from build123d import *

# Parameters (mm, degrees)
SKETCH_1_W          = 10
SKETCH_1_H          = 11.5
SKETCH_1_R          = 1.6
EXTRUDE_1_DEPTH     = 3
SKETCH_2_W          = 15
SKETCH_2_H          = 6
EXTRUDE_2_DEPTH     = 5
FILLET_1_R          = 1
SKETCH_3_W          = 5
SKETCH_3_H          = 5
EXTRUDE_3_DEPTH     = 2
SKETCH_4_W          = 5
SKETCH_4_H          = 3
EXTRUDE_4_DEPTH     = 19.5
SKETCH_5_W          = 5
SKETCH_5_H          = 3.5
EXTRUDE_5_DEPTH     = 3
SKETCH_6_W          = 3
SKETCH_6_H          = 8.5
EXTRUDE_6_DEPTH     = 3
EXTRUDE_7_DEPTH     = 1
SKETCH_8_W          = 3.5
SKETCH_8_H          = 21.5
EXTRUDE_8_DEPTH     = 1
SKETCH_9_W          = 3
SKETCH_9_H          = 8
EXTRUDE_9_DEPTH     = 3.5
EXTRUDE_10_REACH    = 29.208
SKETCH_10_W         = 2.5
SKETCH_10_H         = 3.5
EXTRUDE_11_REACH    = 29.208
SKETCH_11_W         = 3
SKETCH_11_H         = 4
SKETCH_12_W         = 1.5
SKETCH_12_H         = 1.2
CUT_EXTRUDE_1_DEPTH = 2
SKETCH_13_W         = 1
SKETCH_13_H         = 2.5
EXTRUDE_12_DEPTH    = 6.5
SKETCH_14_W         = 1.2
SKETCH_14_H         = 8
EXTRUDE_13_DEPTH    = 6.5
SKETCH_15_W         = 4
SKETCH_15_H         = 4
EXTRUDE_14_DEPTH    = 2.8
FILLET_2_R          = 1
CUT_EXTRUDE_2_REACH = 33.357
SKETCH_16_R         = 1.6
SKETCH_17_W         = 15
SKETCH_17_H         = 5
EXTRUDE_15_DEPTH    = 2
EXTRUDE_16_DEPTH    = 5.5
SKETCH_19_W         = 2
SKETCH_19_H         = 2.8
EXTRUDE_17_DEPTH    = 2
EXTRUDE_18_DEPTH    = 5.5
EXTRUDE_19_DEPTH    = 2.9
EXTRUDE_20_DEPTH    = 0.5
FILLET_3_R          = 2
SKETCH_23_W         = 14.9
SKETCH_23_H         = 1.5
EXTRUDE_21_DEPTH    = 0.5
SKETCH_24_W         = 3
SKETCH_24_H         = 2.8
EXTRUDE_22_DEPTH    = 5
EXTRUDE_23_DEPTH    = 3.2


with BuildPart() as part:
    # 草图1 → 凸台-拉伸1 (new body)
    with BuildSketch(Plane.XY):
        with Locations((1, 0.75)):
            Rectangle(SKETCH_1_W, SKETCH_1_H)
        Circle(SKETCH_1_R, mode=Mode.SUBTRACT)
    extrude(amount=EXTRUDE_1_DEPTH)

    # 草图2 → 凸台-拉伸2 (add)
    with BuildSketch(Plane.XY.offset(3)):
        with Locations((13.5, -2)):
            Rectangle(SKETCH_2_W, SKETCH_2_H)
    extrude(amount=-EXTRUDE_2_DEPTH)

    # 圆角1
    fillet_1_edges = [part.edges().sort_by_distance(p)[0] for p in [
        (-4, 0.75, 0),
    ]]
    fillet(fillet_1_edges, radius=FILLET_1_R)

    # 草图3 → 凸台-拉伸3 (add)
    with BuildSketch(Plane(origin=(0, 1, 0), x_dir=(1, 0, 0), z_dir=(0, 1, 0))):
        with Locations((8.5, -0.5)):
            Rectangle(SKETCH_3_W, SKETCH_3_H)
    extrude(amount=EXTRUDE_3_DEPTH)

    # 草图4 → 凸台-拉伸4 (add)
    with BuildSketch(Plane(origin=(0, 3, 0), x_dir=(1, 0, 0), z_dir=(0, 1, 0))):
        with Locations((8.5, -1.5)):
            Rectangle(SKETCH_4_W, SKETCH_4_H)
    extrude(amount=EXTRUDE_4_DEPTH)

    # 草图5 → 凸台-拉伸5 (add)
    with BuildSketch(Plane(origin=(0, 0, 0), x_dir=(-1, 0, 0), z_dir=(0, 0, -1))):
        with Locations((-8.5, 11.75)):
            Rectangle(SKETCH_5_W, SKETCH_5_H)
    extrude(amount=EXTRUDE_5_DEPTH)

    # 草图6 → 凸台-拉伸6 (add)
    with BuildSketch(Plane.ZY.offset(-6)):
        with Locations((1.5, 18.25)):
            Rectangle(SKETCH_6_W, SKETCH_6_H)
    extrude(amount=EXTRUDE_6_DEPTH)

    # 草图7 → 凸台-拉伸7 (add)
    with BuildSketch(Plane(origin=(0, 0, 0), x_dir=(-1, 0, 0), z_dir=(0, 0, -1))):
        Polygon((-11, 13.5), (-6, 13.5), (-6, 14), (-3, 14), (-3, 22.5), (-11, 22.5), align=None)
    extrude(amount=EXTRUDE_7_DEPTH)

    # 草图8 → 凸台-拉伸8 (add)
    with BuildSketch(Plane.XY.offset(3)):
        with Locations((12.75, 11.75)):
            Rectangle(SKETCH_8_W, SKETCH_8_H)
    extrude(amount=-EXTRUDE_8_DEPTH)

    # 草图9 → 凸台-拉伸9 (add)
    with BuildSketch(Plane(origin=(11, 0, 0), x_dir=(0, 0, -1), z_dir=(1, 0, 0))):
        with Locations((-0.5, 18.5)):
            Rectangle(SKETCH_9_W, SKETCH_9_H)
    extrude(amount=EXTRUDE_9_DEPTH)

    # 凸台-拉伸10: up to this face of the body (flat: up to its plane)
    extrude_10_end = Plane(part.part.faces().sort_by_distance((21, -2, 0.5))[0])
    # 草图10 → 凸台-拉伸10 (add, up to the picked face)
    with BuildSketch(Plane(origin=(11, 0, 0), x_dir=(0, 0, -1), z_dir=(1, 0, 0)), mode=Mode.PRIVATE) as extrude_10_sk1:
        with Locations((-1.75, 2.75)):
            Rectangle(SKETCH_10_W, SKETCH_10_H)
    extrude_10_tool1 = split(extrude(extrude_10_sk1.sketch, amount=EXTRUDE_10_REACH, mode=Mode.PRIVATE), bisect_by=extrude_10_end, keep=Keep.BOTH, mode=Mode.PRIVATE)
    add(extrude_10_tool1.solids().sort_by(Axis((11, 2.75, 1.75), (1, 0, 0)))[0])

    # 凸台-拉伸11: up to this face of the body (flat: up to its plane)
    extrude_11_end = Plane(part.part.faces().sort_by_distance((21, -0.927419355, 0.782258065))[0])
    # 草图11 → 凸台-拉伸11 (add, up to the picked face)
    with BuildSketch(Plane(origin=(11, 0, 0), x_dir=(0, 0, -1), z_dir=(1, 0, 0)), mode=Mode.PRIVATE) as extrude_11_sk1:
        with Locations((-1.5, 12.5)):
            Rectangle(SKETCH_11_W, SKETCH_11_H)
    extrude_11_tool1 = split(extrude(extrude_11_sk1.sketch, amount=EXTRUDE_11_REACH, mode=Mode.PRIVATE), bisect_by=extrude_11_end, keep=Keep.BOTH, mode=Mode.PRIVATE)
    add(extrude_11_tool1.solids().sort_by(Axis((11, 12.5, 1.5), (1, 0, 0)))[0])

    # 草图12 → 切除-拉伸1 (cut)
    with BuildSketch(Plane(origin=(21, 0, 0), x_dir=(0, 0, -1), z_dir=(1, 0, 0))):
        with Locations((-0.75, 13.9)):
            Rectangle(SKETCH_12_W, SKETCH_12_H)
    extrude(amount=-CUT_EXTRUDE_1_DEPTH, mode=Mode.SUBTRACT)

    # 草图13 → 凸台-拉伸12 (add)
    with BuildSketch(Plane(origin=(14.5, 0, 0), x_dir=(0, 0, -1), z_dir=(1, 0, 0))):
        with Locations((-2.5, 9.25)):
            Rectangle(SKETCH_13_W, SKETCH_13_H)
    extrude(amount=EXTRUDE_12_DEPTH)

    # 草图14 → 凸台-拉伸13 (add)
    with BuildSketch(Plane(origin=(14.5, 0, 0), x_dir=(0, 0, -1), z_dir=(1, 0, 0))):
        with Locations((-2.4, 18.5)):
            Rectangle(SKETCH_14_W, SKETCH_14_H)
    extrude(amount=EXTRUDE_13_DEPTH)

    # 草图15 → 凸台-拉伸14 (add)
    with BuildSketch(Plane(origin=(0, 0, 1.8), x_dir=(-1, 0, 0), z_dir=(0, 0, -1))):
        with Locations((-16.5, 16.5)):
            Rectangle(SKETCH_15_W, SKETCH_15_H)
    extrude(amount=EXTRUDE_14_DEPTH)

    # 圆角2
    fillet_2_edges = [part.edges().sort_by_distance(p)[0] for p in [
        (14.5, 18.5, 0.4),
    ]]
    fillet(fillet_2_edges, radius=FILLET_2_R)

    # 草图16 → 切除-拉伸2 (cut, up to next)
    with BuildSketch(Plane.XY.offset(3), mode=Mode.PRIVATE) as cut_extrude_2_sk1:
        with Locations((6.75, 19)):
            Circle(SKETCH_16_R)
    cut_extrude_2_tool1 = extrude(cut_extrude_2_sk1.sketch, amount=-CUT_EXTRUDE_2_REACH, mode=Mode.PRIVATE) & part.part
    add(cut_extrude_2_tool1.solids().sort_by_distance((6.75, 19, 3))[0], mode=Mode.SUBTRACT)

    # 草图17 → 凸台-拉伸15 (add)
    with BuildSketch(Plane.XZ.offset(5)):
        with Locations((13.5, 0.5)):
            Rectangle(SKETCH_17_W, SKETCH_17_H)
    extrude(amount=EXTRUDE_15_DEPTH)

    # 草图18 → 凸台-拉伸16 (add)
    with BuildSketch(Plane(origin=(21, 0, 0), x_dir=(0, 0, -1), z_dir=(1, 0, 0))):
        Polygon((0, 13.3), (-1.5, 13.3), (-1.5, 14.5), (-1.8, 14.5), (-1.8, 22.5), (-3, 22.5), (-3, 8), (-2, 8), (-2, 10.5), (0, 10.5), align=None)
    extrude(amount=EXTRUDE_16_DEPTH)

    # 草图19 → 凸台-拉伸17 (add)
    with BuildSketch(Plane(origin=(0, 0, 0), x_dir=(-1, 0, 0), z_dir=(0, 0, -1))):
        with Locations((-25.5, 11.9)):
            Rectangle(SKETCH_19_W, SKETCH_19_H)
    extrude(amount=EXTRUDE_17_DEPTH)

    # 草图20 → 凸台-拉伸18 (add)
    with BuildSketch(Plane(origin=(21, 0, 0), x_dir=(0, 0, -1), z_dir=(1, 0, 0))):
        Polygon((0.5, -3), (-3, -3), (-3, 4.5), (0.5, 4.5), (0.5, 1), (2, 1), (2, -3), align=None)
    extrude(amount=EXTRUDE_18_DEPTH)

    # 草图21 → 凸台-拉伸19 (add)
    with BuildSketch(Plane(origin=(26.5, 0, 0), x_dir=(0, 0, -1), z_dir=(1, 0, 0))):
        Polygon((-3, -3), (2, -3), (2, 1), (0.5, 1), (0.5, 4.5), (-3, 4.5), align=None)
        Polygon((-2, 10.5), (2, 10.5), (2, 13.3), (-1.5, 13.3), (-1.5, 14.5), (-1.8, 14.5), (-1.8, 22.5), (-3, 22.5), (-3, 8), (-2, 8), align=None)
    extrude(amount=EXTRUDE_19_DEPTH)

    # 草图22 → 凸台-拉伸20 (add)
    with BuildSketch(Plane(origin=(0, 0, 2), x_dir=(-1, 0, 0), z_dir=(0, 0, -1))):
        Polygon((-11, 10.5), (-29.4, 10.5), (-29.4, 8), (-14.5, 8), (-14.5, 4.5), (-11, 4.5), align=None)
    extrude(amount=EXTRUDE_20_DEPTH)

    # 圆角3
    fillet_3_edges = [part.edges().sort_by_distance(p)[0] for p in [
        (25.2, -3, 3),
    ]]
    fillet(fillet_3_edges, radius=FILLET_3_R)

    # 草图23 → 凸台-拉伸21 (add)
    with BuildSketch(Plane.XZ.offset(-8)):
        with Locations((21.95, 2.25)):
            Rectangle(SKETCH_23_W, SKETCH_23_H)
    extrude(amount=EXTRUDE_21_DEPTH)

    # 草图24 → 凸台-拉伸22 (add)
    with BuildSketch(Plane(origin=(29.4, 0, 0), x_dir=(0, 0, -1), z_dir=(1, 0, 0))):
        with Locations((0.5, 11.9)):
            Rectangle(SKETCH_24_W, SKETCH_24_H)
    extrude(amount=EXTRUDE_22_DEPTH)

    # 草图25 → 凸台-拉伸23 (add)
    with BuildSketch(Plane(origin=(0, 22.5, 0), x_dir=(1, 0, 0), z_dir=(0, 1, 0))):
        Polygon((9.9, 1), (9.9, -3), (29.4, -3), (29.4, -1.8), (14.5, -1.8), (14.5, 1), align=None)
    extrude(amount=EXTRUDE_23_DEPTH)


solid = part.part
Can you work these out from the model? Positions are in its coordinate system, mm. A direction names the side the tool comes from. Round coordinates to 2 decimals unless told otherwise and drop trailing zeros. Order: outer loops, then holes, each group sorted by start corner. A loop starts at its lowest first (then second) coordinate and runs counter-clockwise, first axis right, second up. Notation, with made-up numbers: M 4.25,70.5 L 53.25,70.5 A26 cw 53.25,105.5 Z; hole C 38,80.25 d11. An arc over 180 degrees is marked long. Use a Markdown table: item, result.
1) Imagine slicing it at A-A (x = 19.5). List the corners of the cut face in (y, z) for me.
Geometry says:
| item | result |
|---|---|
| outline | M -7,-2 L 1,-2 L 1,0.5 L 4.5,0.5 L 4.5,3 L -7,3 Z; M 7.5,1.5 L 10.5,1.5 L 10.5,0 L 13.3,0 L 13.3,1.5 L 14.5,1.5 L 14.5,1.8 L 25.7,1.8 L 25.7,3 L 7.5,3 Z |
2) Imagine slicing it at C-C (x = 4). List the corners of the cut face in (y, z) for me, then the cut area to 3 significant figures.
Geometry says:
| item | result |
|---|---|
| outline | M -5,0 L 6.5,0 L 6.5,3 L -5,3 Z; M 14,-1 L 22.5,-1 L 22.5,3 L 14,3 Z |
| area | 68.5 mm² |
3) If I drill on line 1 along Y through (x, z) = (0, 0.7); line 2 along Y through (x, z) = (8, -1.6); line 3 along X through (y, z) = (6, 2.55), over which ranges is the centre line in solid material (lowest first)?
Geometry says:
| item | result |
|---|---|
| line 1 | y = -5 to -1.6, 1.6 to 6.5 |
| line 2 | y = -7 to 3, 10 to 13.5 |
| line 3 | x = -4 to 14.5 |
4) Imagine slicing it at D-D (y = 15). List the corners of the cut face in (x, z) for me.
Geometry says:
| item | result |
|---|---|
| outline | M 3,-1 L 18.5,-1 L 18.5,1.8 L 29.4,1.8 L 29.4,3 L 3,3 Z |
5) On a 3-axis mill with a long thin cutter (end or side, diameter ignored), from which of +Z, -Z, +X, -X, +Y, -Y can I reach the whole of each face in a straight line? I mean faces 4 (the face through (6, 10, 1)), 5 (the face through (25, 3, -0.5)), 6 (the face through (11, 7.8, 0.3)), 7 (the face through (15, -2, -2)), 8 (the face through (11, 18, -1)). Say none if no direction works.
Geometry says:
| item | result |
|---|---|
| face 4 | +Z, -Z, -X |
| face 5 | -Z, +X |
| face 6 | -Z |
| face 7 | -Z, +X, -X, -Y |
| face 8 | -Z, +X, -X, +Y |
6) Imagine slicing it at B-B (y = 0). List the corners of the cut face in (x, z) for me, then the cut area to 3 significant figures.
Geometry says:
| item | result |
|---|---|
| outline | M -4,1 A1 ccw -3,0 L -1.6,0 L -1.6,3 L -4,3 Z; M 1.6,0 L 6,0 L 6,-2 L 29.4,-2 L 29.4,3 L 1.6,3 Z |
| area | 137 mm² |
7) If we mould it in two halves opening along Y, with no side actions, what happens to faces 1 (the face through (14.5, 6, 2)), 2 (the face through (-4, 1, 2)), 3 (the face through (9, 13.5, -2))? For each: +Y half, -Y half, draft (parallel to the pull), parting line (faces both ways), or undercut.
Geometry says:
| item | result |
|---|---|
| face 1 | undercut |
| face 2 | draft |
| face 3 | +Y half |
8) I'm going to push flat-ended pins straight in: P1, Ø3, axis at x = 16, y = 0, coming from the -Z side; P2, Ø1.3, axis at y = 14, z = 1, coming from the +X side; P3, Ø5, axis at x = 6.75, y = 19, coming from the -Z side. Where does each tip first touch, or does it pass through?
Geometry says:
| item | result |
|---|---|
| P1 | stops at z = -2 |
| P2 | stops at x = 29.4 |
| P3 | stops at z = -1 |
